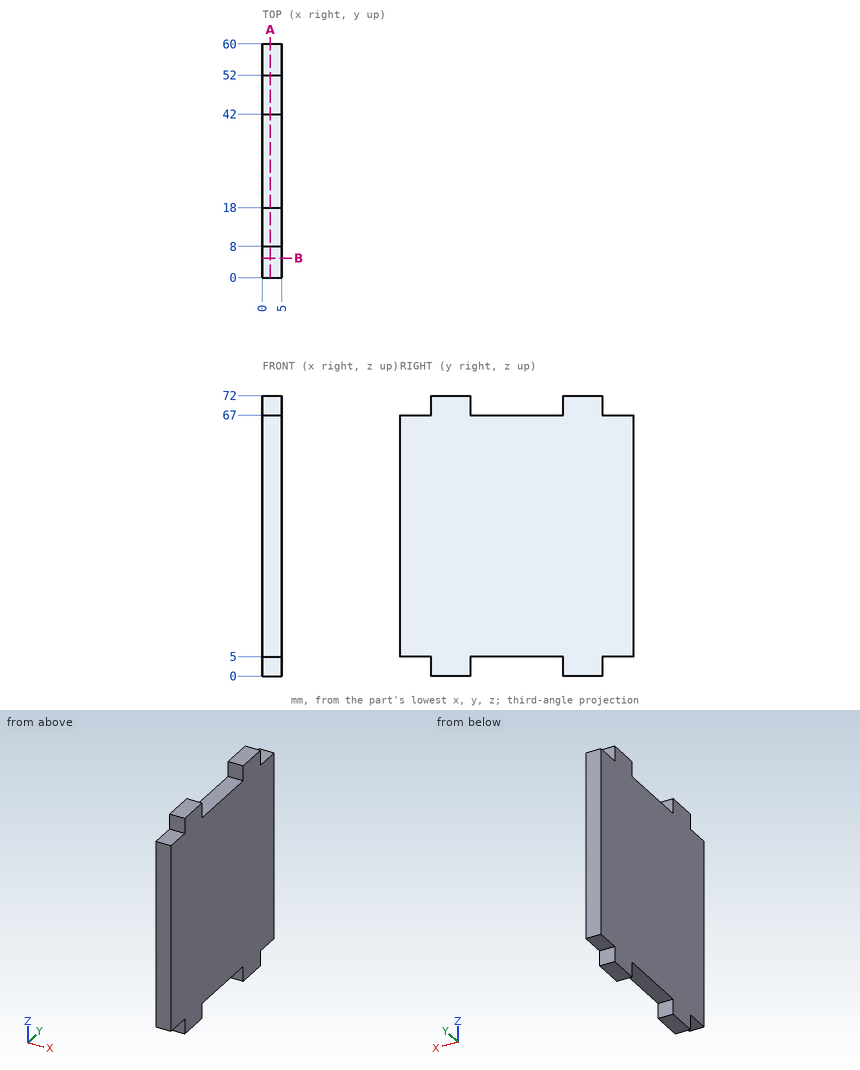
Print and shaded views of the part. All mm, measured from the part's lowest x, y and z. Round coordinates to 2 decimals unless told otherwise and drop trailing zeros. Write each loop counter-clockwise with the first axis right and the second up, starting at its lowest first coordinate (ties: lowest second). Pieces come first, ordered by that corner, then holes. Notation, with made-up numbers: (16.5, -37) - (58.5, -37) arc R16 cw to (58.5, -32) - close; hole circle Ø7 at (80.5, 6.25). An arc over 180 degrees is marked (long way). Use CSV: the item, a comma, the result in double quotes. Start each with the question number.
Item 1: Drill centre lines: L1, parallel to Y at x = 3.1, z = 69; L2, parallel to Z at x = 0.95, y = 28. Where is each one in solid material? Low to high. Write a range as [from, to].
Item 2: Band-saw the part on A-A (x = 2.05). Write the cut outline in (y, z), and give its area (3 significant figures).
Item 3: Pin check, flat tips, straight feed: P1, Ø1.5, axis at x = 2, z = 70.5, coming from the -Y side; P2, Ø1.5, axis at x = 2.5, y = 57, coming from the +Z side; P3, Ø2.5, axis at x = 1.5, y = 4.5, coming from the -Z side. Stop position of each tip, or through.
Item 4: Band-saw the part on B-B (y = 5). Write the cut outline in (x, z), and give its area (3 significant figures).
Checked values:
1,L1,"y = [8, 18], [42, 52]"
1,L2,"z = [5, 67]"
2,outline,"(0, 5) - (8, 5) - (8, 0) - (18, 0) - (18, 5) - (42, 5) - (42, 0) - (52, 0) - (52, 5) - (60, 5) - (60, 67) - (52, 67) - (52, 72) - (42, 72) - (42, 67) - (18, 67) - (18, 72) - (8, 72) - (8, 67) - (0, 67) - close"
2,area,"3,920 mm²"
3,P1,"stops at y = 8"
3,P2,"stops at z = 67"
3,P3,"stops at z = 5"
4,outline,"(0, 5) - (5, 5) - (5, 67) - (0, 67) - close"
4,area,"310 mm²"
